Can you work these out from the model? Positions are in its coordinate system, mm. Give positions to 0.01 mm unless a question says otherwise; leave off trailing zeros. Write each loop counter-clockwise with the first axis right and the second up, starting at its lowest first coordinate (ties: lowest second). Pieces come first, ordered by that corner, then holes.
1. Suppose I cut it at B-B (y = 171.45). Please give me the cut outline in (x, z) (3 decimals).
2. Suppose I cut it at A-A (x = 152.4). Please give me the cut outline in (y, z) (3 decimals), and give its area (3 significant figures).
3. If I drill on probe 1 along Y at (x, z) = (152, 0.55); probe 2 along X at (y, z) = (6.35, 1.6), over which ranges is the centre line in solid material (lowest first)?
4. I'm going to push a flat-ended pin straight in: pin 1 (1.5 mm diameter, centred on x = 76.5, y = 58, fed in from -Z). Where does the tip first touch, or does it pass through?
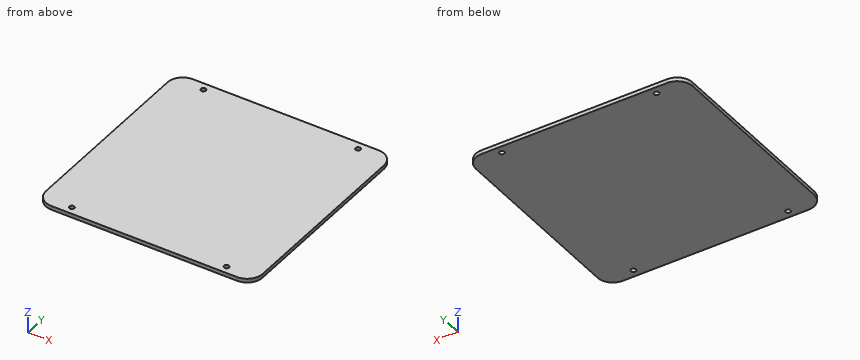
Autodesk Fusion 360 part; units mm, degrees
sketch "Sketch1" plane through (0, 0, 0) normal (0, 0, 1) x (1, 0, 0)
  line L0 (0, 0) -> (177.8, 0)
  line L1 (177.8, 0) -> (177.8, 177.8)
  line L2 (177.8, 177.8) -> (0, 177.8)
  line L3 (0, 177.8) -> (0, 0)
  dimension "d2" = 177.8
  dimension "d3" = 177.8
extrude "Extrude1" add sketch "Sketch1" along normal blind 3.175
fillet "Fillet1" radius 12.7 4 edges at (177.8, 0, 1.5875) (0, 0, 1.5875) (177.8, 177.8, 1.5875) (0, 177.8, 1.5875)
sketch "Sketch2" plane through (0, 0, 3.175) normal (0, 0, 1) x (-1, 0, 0)
  arc A0 (-12.7, -177.8) -> (0, -165.1) centre (-12.7, -165.1) ccw
  line L0 (0, -165.1) -> (0, -12.7)
  arc A1 (0, -12.7) -> (-12.7, 0) centre (-12.7, -12.7) ccw
  line L1 (-12.7, 0) -> (-165.1, 0)
  arc A2 (-165.1, 0) -> (-177.8, -12.7) centre (-165.1, -12.7) ccw
  line L2 (-177.8, -12.7) -> (-177.8, -165.1)
  arc A3 (-177.8, -165.1) -> (-165.1, -177.8) centre (-165.1, -165.1) ccw
  line L3 (-165.1, -177.8) -> (-12.7, -177.8)
  line L4 (-25.4, -171.45) -> (-152.4, -171.45) construction
  line L5 (-152.4, -171.45) -> (-152.4, -6.35) construction
  line L6 (-152.4, -6.35) -> (-25.4, -6.35) construction
  line L7 (-25.4, -6.35) -> (-25.4, -171.45) construction
  line L8 (-152.4, -100.0288) -> (-177.8, -100.0288) construction
  line L9 (-25.4, -101.0393) -> (0, -101.0393) construction
  line L10 (-70.6928, -171.45) -> (-70.6928, -177.8) construction
  line L11 (-68.6718, -6.35) -> (-68.6718, 0) construction
  circle A4 centre (-152.4, -6.35) radius 2.05
  dimension "d8" = 25.4
  dimension "d9" = 6.35
  dimension "d10" = 4.1
extrude "Extrude2" cut sketch "Sketch2" against normal through all contours A4
pattern_linear "R-Pattern1" count 2 spacing 127 along (-1, 0, 0) count 2 spacing 165.1 along (0, 1, 0) of "Extrude2"
equation "side = 7 in"
equation "d2 = side"
equation "d3 = side"
equation "d4 = ( 1 / 8 ) * 1 in"
Checks:
1. outline: (1.701, 0) - (23.35, 0) - (23.35, 3.175) - (1.701, 3.175) - close; (27.45, 0) - (150.35, 0) - (150.35, 3.175) - (27.45, 3.175) - close; (154.45, 0) - (176.099, 0) - (176.099, 3.175) - (154.45, 3.175) - close
2. outline: (0, 0) - (4.3, 0) - (4.3, 3.175) - (0, 3.175) - close; (8.4, 0) - (169.4, 0) - (169.4, 3.175) - (8.4, 3.175) - close; (173.5, 0) - (177.8, 0) - (177.8, 3.175) - (173.5, 3.175) - close
2. area: 538 mm2
3. probe 1: y = 0 to 4.34, 8.36 to 169.44, 173.46 to 177.8
3. probe 2: x = 1.7 to 23.35, 27.45 to 150.35, 154.45 to 176.1
4. pin 1: stops at z = 0
